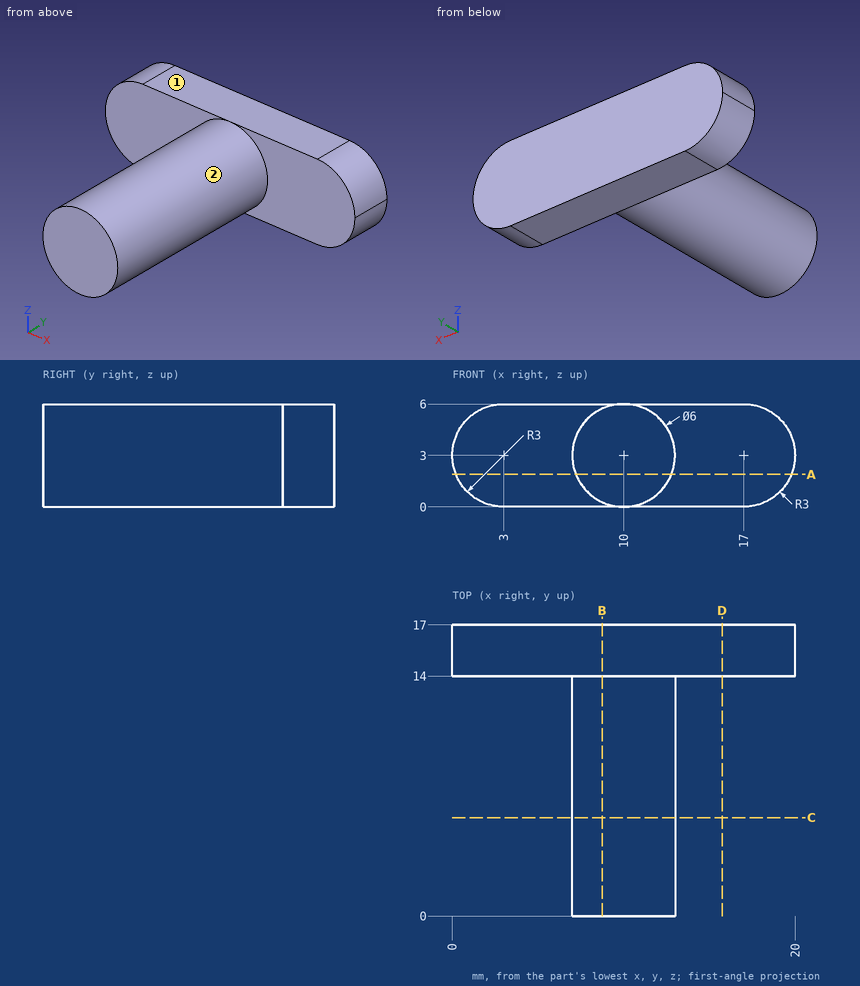
Drawing for the job (mm, zero at the part's lowest x, y, z). A direction names the side the tool comes from. Round coordinates to 2 decimals unless told otherwise and drop trailing zeros. Order: outer loops, then holes, each group sorted by start corner. A loop starts at its lowest first (then second) coordinate and runs counter-clockwise, first axis right, second up.
Item 1: Tool access for the marked faces 1 and 2: list every direction of +Z, -Z, +X, -X, +Y, -Y with a clear straight run to the whole face (end or side of a thin tool).
Item 2: Probe line 1 along Y through (x, z) = (3, 2.9); line 2 along X through (y, z) = (12.25, 3); line 3 along X through (y, z) = (6, 4.75). List the from-to ranges inside material, lowest first.
Item 3: Saw through at C-C on y = 5.75. Write the cut outline in (x, z), then the cut area to 3 significant figures.
Item 4: Saw through at A-A on z = 1.9. Write the cut outline in (x, y), then the cut area to 3 significant figures.
Item 5: Saw through at B-B on x = 8.75. Write the cut outline in (y, z), then the cut area to 3 significant figures.
Item 6: Saw through at D-D on x = 15.75. Write the cut outline in (y, z).
Item 7: Pin check, flat tips, straight feed: pin 1 (3 mm diameter, centred on x = 13.5, y = 7.5, fed in from -Z); pin 2 (1 mm diameter, centred on y = 4, z = 1.5, fed in from +X); pin 3 (5 mm diameter, centred on x = 15, y = 7, fed in from -Z); pin 4 (1.8 mm diameter, centred on x = 7.5, z = 3, fed in from -Y). Stop position of each tip, or through.
Reported:
1. face 1: +Z, +X, -X, +Y, -Y
1. face 2: -Y
2. line 1: y = 14 to 17
2. line 2: x = 7 to 13
2. line 3: x = 7.56 to 12.44
3. outline: circle Ø6 at (10, 3)
3. area: 28.3 mm2
4. outline: (0.21, 14) - (7.21, 14) - (7.21, 0) - (12.79, 0) - (12.79, 14) - (19.79, 14) - (19.79, 17) - (0.21, 17) - close
4. area: 137 mm2
5. outline: (0, 0.27) - (14, 0.27) - (14, 0) - (17, 0) - (17, 6) - (14, 6) - (14, 5.73) - (0, 5.73) - close
5. area: 94.4 mm2
6. outline: (14, 0) - (17, 0) - (17, 6) - (14, 6) - close
7. pin 1: stops at z = 0.76
7. pin 2: stops at x = 12.83
7. pin 3: stops at z = 1.34
7. pin 4: stops at y = 0
